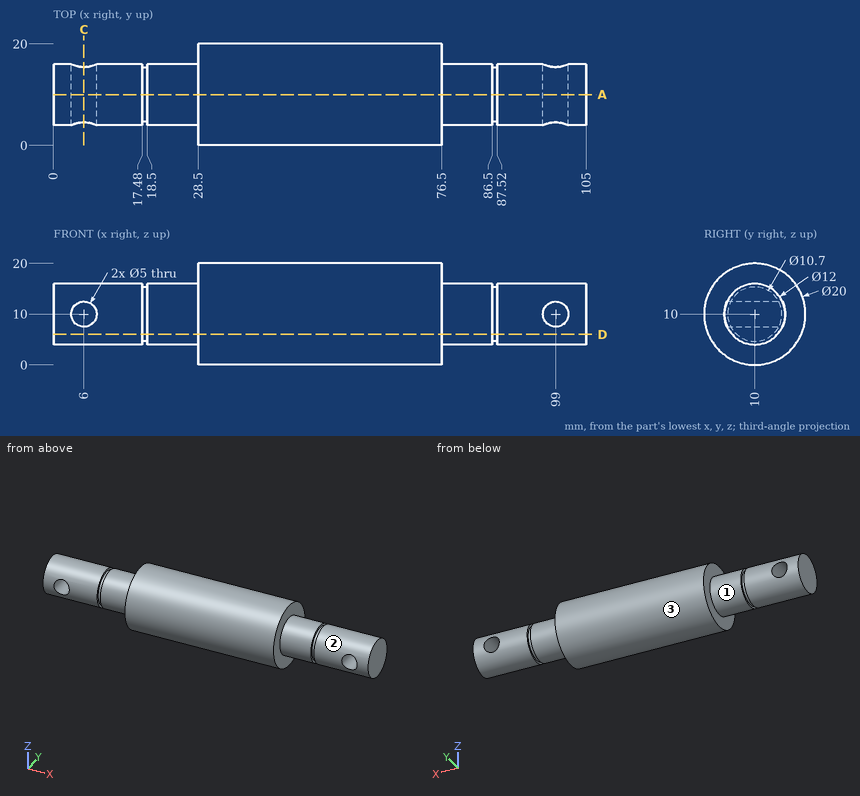
Part print with two shaded views. Sizes in mm from the minimum x, y, z corner. A direction names the side the tool comes from. Round coordinates to 2 decimals unless told otherwise and drop trailing zeros. Write each loop counter-clockwise with the first axis right and the second up, starting at its lowest first coordinate (ties: lowest second). Pieces come first, ordered by that corner, then holes. Notation, with made-up numbers: M 13.5,-13.5 L 53.5,-13.5 A11 ccw 53.5,6.5 Z; hole C -31.75,4.25 d11. An arc over 180 degrees is marked long. Put each result on its own line as item: value. Start each with the question number.
1) Saw through at C-C, the plane x = 6. Write the cut outline in (y, z).
2) 3-axis set-ups, long thin cutter, end or side, ignore diameter. For the marked faces 1, 2 and 3: which of +Z, -Z, +X, -X, +Y, -Y reach the whole face in a straight line?
3) Saw through at D-D, the plane z = 6. Write the cut outline in (x, y).
4) Pin check, flat tips, straight feed: pin 1 Ø10 at (x, y) = (40.5, 12) entering from +Z; pin 2 Ø6 at (x, z) = (6, 10) entering from -Y; pin 3 Ø3 at (y, z) = (4, 15.5) entering from -X; pin 4 Ø1 at (y, z) = (2.5, 9) entering from +X. Stop position of each tip, or through.
5) Saw through at A-A, the plane y = 10. Count the separate pieces of the cut face and the enclosed holes in it, and give its area (3 significant figures).
6) Drill centre lines: probe 1 along X at (y, z) = (8.5, 10); probe 2 along Z at (x, y) = (6, 10.25); probe 3 along X at (y, z) = (9.5, 11). Where is each one in solid material? Low to high. Write a range as [from, to].
Resolved:
1. outline: M 4.55,7.5 A6 ccw 15.45,7.5 Z; M 4.55,12.5 L 15.45,12.5 A6 ccw Z
2. face 1: -X
2. face 2: +X
2. face 3: +X, -X
3. outline: M 0,5.53 L 17.48,5.53 L 17.48,6.45 L 18.5,6.45 L 18.5,5.53 L 28.5,5.53 L 28.5,0.83 L 76.5,0.83 L 76.5,5.53 L 86.5,5.53 L 86.5,6.45 L 87.52,6.45 L 87.52,5.53 L 105,5.53 L 105,14.47 L 87.52,14.47 L 87.52,13.55 L 86.5,13.55 L 86.5,14.47 L 76.5,14.47 L 76.5,19.17 L 28.5,19.17 L 28.5,14.47 L 18.5,14.47 L 18.5,13.55 L 17.48,13.55 L 17.48,14.47 L 0,14.47 Z
4. pin 1: z = 20
4. pin 2: y = 4
4. pin 3: x = 28.5
4. pin 4: x = 76.5
5. separate pieces: 1
5. enclosed holes: 2
5. area: 1,600 mm²
6. probe 1: [0, 3.5], [8.5, 96.5], [101.5, 105]
6. probe 2: [4.01, 7.5], [12.5, 15.99]
6. probe 3: [0, 3.71], [8.29, 96.71], [101.29, 105]
